Input: part model. Units: mm. Frame: model coordinates. A direction names the side the tool comes from. Give positions to 0.01 mm unless a question says otherwise; leave off trailing zeros. Loops run counter-clockwise (first coordinate to the right, second up) from the corner with the lowest first, then second, coordinate; pieces in that order, holes last. Notation, with made-up numbers: M 15.5,85 L 50.5,85 A13 ccw 50.5,102 Z; hole C 36,-39.75 d5. An arc over 180 degrees is marked long. Answer as a JSON object with one key per item and string values. Group by question number.
1) Ray query, L1, parallel to Z at x = 0, y = -5.75; L2, parallel to Y at x = -2.2, z = -0.4; L3, parallel to Z at x = 0.6, y = 0.5. Return the intervals inside material, ascending.
2) Access query for faces 5 (the flat face through (1, -7.62, -2)), 6 (the flat face through (0, 11.43, 0)). Directions: +Z, -Z, +X, -X, +Y, -Y. A direction counts if a zero-diameter tool reaches every point of the face in a straight line with its end or side. Return the directions, or none.
3) Draft query along X for faces 1 (the flat face through (0, 11.176, 0)), 2 (the cylindrical face through (2.726, -0.107, 0.858)), 3 (the flat face through (1, 7.62, -2)), 4 (the cylindrical face through (-0.385, -0.285, -1.736)). Return one class per face: +X half, -X half, draft (parallel to the pull), parting line (faces both ways), or undercut.
4) Section query D-D on y = -9.25. Return loops of the section in (x, z) (3 decimals).
5) First-contact query: P1, Ø1.5, axis at x = 2, y = 1.5, coming from the -Z side; P2, Ø1.1, axis at x = -0.5, z = -1, coming from the -Y side; P3, Ø2, axis at y = -4.5, z = -2, coming from the -X side. Flat tips, straight axial feed; report the tip coordinate or a pass-through.
6) Section query B-B on y = -0.5. Return loops of the section in (x, z) (1 decimal).
from build123d import *

# Parameters (mm, degrees)
F0_R     = 2.8575
F1_DEPTH = 7.62
F2_R     = 1.905
F3_DEPTH = 11.43
F4_R     = 1.778
F5_DEPTH = 22.606


with BuildPart() as f1:
    # F0 (on Front) → F1 (new body, symmetric)
    with BuildSketch(Plane.XZ):
        Circle(F0_R)
    extrude(amount=F1_DEPTH, both=True)

    # F2 (on Front) → F3 (join, symmetric)
    with BuildSketch(Plane.XZ):
        Circle(F2_R)
    extrude(amount=F3_DEPTH, both=True)

    # F4 (on face) → F5 (cut)
    with BuildSketch(Plane.XZ.offset(11.43)):
        Circle(F4_R)
    extrude(amount=-F5_DEPTH, mode=Mode.SUBTRACT)


solid = f1.part
Output:
{
 "1": {"L1": "z = -2.86 to -1.78, 1.78 to 2.86", "L2": "y = -7.62 to 7.62", "L3": "z = -2.79 to -1.67, 1.67 to 2.79"},
 "2": {"face 5": "-Y", "face 6": "+Z, -Z, +X, -X, +Y"},
 "3": {"face 1": "undercut", "face 2": "parting line", "face 3": "draft", "face 4": "undercut"},
 "4": {"outline": "C 0,0 d3.81; hole C 0,0 d3.556"},
 "5": {"P1": "stops at z = -2.57", "P2": "stops at y = 11.18", "P3": "stops at x = -2.68"},
 "6": {"outline": "C 0,0 d5.7; hole C 0,0 d3.6"}
}
